The listing builds one solid part. Answer for the finished solid, in the listing's coordinates (mm). Face numbers are marked on the shaded views. A direction names the side the tool comes from. Coordinates: 2 decimals unless noted, no trailing zeros. Write each loop counter-clockwise with the first axis right and the second up, starting at its lowest first coordinate (ties: lowest second). Pieces come first, ordered by that corner, then holes.
from build123d import *

# Parameters (mm, degrees)
F0_W     = 540
F0_H     = 80
F1_DEPTH = 10
F2_W     = 540
F2_H     = 10
F3_DEPTH = 70
F4_R     = 11
F5_DEPTH = 80.001
F6_R     = 9
F7_DEPTH = 80.001


with BuildPart() as f1:
    # F0 (on Front) → F1 (new body)
    with BuildSketch(Plane.XZ):
        with Locations((270, 40)):
            Rectangle(F0_W, F0_H)
    extrude(amount=F1_DEPTH)

    # F2 (on face) → F3 (join)
    with BuildSketch(Plane.XZ.offset(10)):
        with Locations((270, 75)):
            Rectangle(F2_W, F2_H)
    extrude(amount=F3_DEPTH)

    # F4 (on face) → F5 (cut, through all)
    with BuildSketch(Plane(origin=(0, 0, 0), x_dir=(-1, 0, 0), z_dir=(0, 1, 0))):
        with Locations((-505, 35)):
            Circle(F4_R)
        with Locations((-387.5, 35)):
            Circle(F4_R)
        with Locations((-270, 35)):
            Circle(F4_R)
        with Locations((-152.5, 35)):
            Circle(F4_R)
        with Locations((-35, 35)):
            Circle(F4_R)
    extrude(amount=-F5_DEPTH, mode=Mode.SUBTRACT)

    # F6 (on face) → F7 (cut, through all)
    with BuildSketch(Plane.XY.offset(80)):
        with Locations((26, -45)):
            Circle(F6_R)
        with Locations((514, -45)):
            Circle(F6_R)
    extrude(amount=-F7_DEPTH, mode=Mode.SUBTRACT)


solid = f1.part
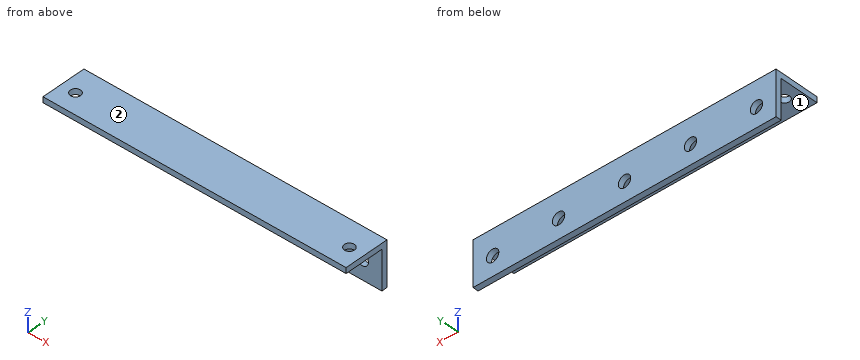
Q1. Find the intervals of material crossed by probe 1 along Z at (x, y) = (152.5, -5); probe 2 along Y at (x, z) = (514, 72.5); probe 3 along Y at (x, z) = (212, 34), in increasing order.
Answers below:
probe 1: z = 0 to 24, 46 to 80
probe 2: y = -80 to -54, -36 to 0
probe 3: y = -10 to 0
Q2. Given pin 1 (1.5 mm diameter, centred on x = 278, y = -61.5, fed in from -Z); pin 2 (11 mm diameter, centred on x = 26, y = -45, fed in from +Z), each flat-ended and moving along its own axis, determine where each tip first touches the part or whether it passes through.
Answers below:
pin 1: stops at z = 70
pin 2: passes through
Q3. Which of the six approach directions +Z, -Z, +X, -X, +Y, -Y give full straight-line access (tool end or side, diameter ignored) to the marked faces 1 and 2?
Answers below:
face 1: -Z, +X, -X, -Y
face 2: +Z, +X, -X, +Y, -Y
Q4. The part is cut by section C-C, the plane z = 35. Write down the section's boundary in (x, y).
Answers below:
outline: (0, -10) - (24, -10) - (24, 0) - (0, 0) - close; (46, -10) - (141.5, -10) - (141.5, 0) - (46, 0) - close; (163.5, -10) - (259, -10) - (259, 0) - (163.5, 0) - close; (281, -10) - (376.5, -10) - (376.5, 0) - (281, 0) - close; (398.5, -10) - (494, -10) - (494, 0) - (398.5, 0) - close; (516, -10) - (540, -10) - (540, 0) - (516, 0) - close
Q5. The part is cut by section B-B, the plane x = 387.5. Write down the section's boundary in (y, z).
Answers below:
outline: (-80, 70) - (-10, 70) - (-10, 46) - (0, 46) - (0, 80) - (-80, 80) - close; (-10, 0) - (0, 0) - (0, 24) - (-10, 24) - close
Q6. The part is cut by section D-D, the plane x = 124. Write down the section's boundary in (y, z), then the cut area to 3 significant figures.
Answers below:
outline: (-80, 70) - (-10, 70) - (-10, 0) - (0, 0) - (0, 80) - (-80, 80) - close
area: 1,500 mm2
Q7. The part is cut by section A-A, the plane y = -45. Write down the section's boundary in (x, z), then the cut area to 3 significant figures.
Answers below:
outline: (0, 70) - (17, 70) - (17, 80) - (0, 80) - close; (35, 70) - (505, 70) - (505, 80) - (35, 80) - close; (523, 70) - (540, 70) - (540, 80) - (523, 80) - close
area: 5,040 mm2
